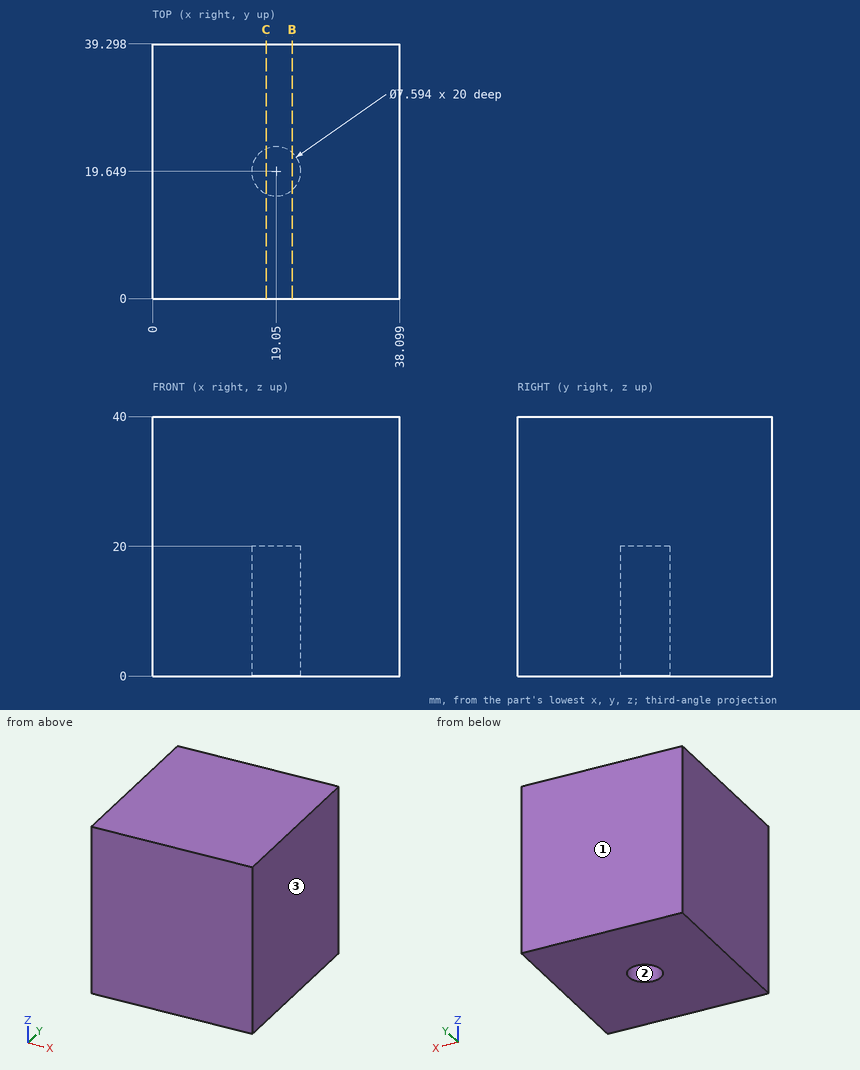
Print and shaded views of the part. All mm, measured from the part's lowest x, y and z. Round coordinates to 2 decimals unless told otherwise and drop trailing zeros. Loops run counter-clockwise (first coordinate to the right, second up) from the corner with the lowest first, then second, coordinate; pieces in that order, holes last. Notation, with made-up numbers: M 10.5,45.5 L 65.5,45.5 A29 ccw 65.5,66.5 Z; hole C 80,17 d7. An arc over 180 degrees is marked long. One line per question, with ' | ' between items.
1) Mould opens along Y. For the marked faces 1, 2 and 3 say: +Y half, -Y half, draft (parallel to the pull), parting line (faces both ways), or undercut.
Solved:
face 1: +Y half | face 2: undercut | face 3: draft
2) Band-saw the part on C-C (x = 17.5). Give the cut face in (y, z) (1 decimal).
Solved:
outline: M 0,0 L 16.2,0 L 16.2,20 L 23.1,20 L 23.1,0 L 39.3,0 L 39.3,40 L 0,40 Z
3) Drill centre lines: line 1 along Y through (x, z) = (17, 19) (1 decimal); line 2 along X through (y, z) = (16.5, 15) (1 decimal). Where is each one in solid material? Low to high.
Solved:
line 1: y = 0 to 16.5, 22.8 to 39.3 | line 2: x = 0 to 16.9, 21.2 to 38.1
4) Flat gauge pin, fed straight in: pin 1 (2.5 mm diameter, centred on x = 19.5, y = 19, fed in from -Z). Where does the tip first touch, or does it go through?
Solved:
pin 1: stops at z = 20
5) Band-saw the part on B-B (x = 21.5). Give the cut face in (y, z).
Solved:
outline: M 0,0 L 16.75,0 L 16.75,20 L 22.55,20 L 22.55,0 L 39.3,0 L 39.3,40 L 0,40 Z
